Verification items for the finished model (mm, model axes). Face numbers are marked on the shaded views. Give positions to 0.01 mm unless a question says otherwise; leave off trailing zeros. Loops run counter-clockwise (first coordinate to the right, second up) from the corner with the lowest first, then second, coordinate; pieces in that order, holes last. Notation, with made-up numbers: (80.25, 76.25) -> (118.25, 76.25) arc R21 cw to (118.25, 93.25) -> close; hole circle Ø9 at (-35, 55). An arc over 180 degrees is marked (long way). Answer in a Markdown table with one row per item. Add a question column.
Q1. Section check B-B on z = 5. Give the number of separate pieces and of enclosed holes in the cut face, and give its area (3 significant figures).
Q2. Section check C-C on x = 1.5. Enter the section's corners in (y, z).
Q3. Material ranges on probe 1 along Y at (x, z) = (-6, -20); probe 2 along X at (y, z) = (-5.5, 2); probe 3 along Z at (x, y) = (-9, -5.5), recorded low to high.
Q4. Gauge pin test, flat ends, axial feed: P1, Ø1.4, axis at x = 10.5, y = -5, coming from the -Z side; P2, Ø0.6, axis at x = -10.5, y = -3, coming from the -Z side; P3, Ø1.5, axis at x = 13.5, y = -2.5, coming from the +Z side. Record the tip position at first contact, or that the pin passes through.
Q5. Release check for a two-part mould opening along X. For the marked faces 1, 2 and 3 record: pulls with the +X half, pulls with the -X half, needs draft (parallel to the pull), parting line crosses it, or undercut.
Q6. Section check A-A on z = -5.5. Enter the section's corners in (x, y), and give its area (3 significant figures).
```python
from build123d import *

# Parameters (mm, degrees)
F0_R     = 25.4
F1_DEPTH = 6.35
F3_DEPTH = 6.604
F4_DEPTH = 6.604


# Not quite as in the source:
# - the program builds the solid bodies; features that only make, move or delete a surface that nothing else refers to are left out


with BuildPart() as f1:
    # F0 (on Front) → F1 (new body)
    with BuildSketch(Plane.XZ):
        Circle(F0_R)
        with BuildLine():
            Line((-11.384175581, -2.9492764653), (-13.375339268, -2.9492764653))
            Line((-13.375339268, -2.9492764653), (-15.3665029551, -12.3323677108))
            Line((-15.3665029551, -12.3323677108), (-20.4675217554, -12.3323677108))
            Line((-20.4675217554, -12.3323677108), (-15.3022718684, 12.1236185417))
            Line((-15.3022718684, 12.1236185417), (-9.296665264, 12.1236185417))
            add(Edge.make_bspline(
                [(-9.296665264, 12.1236185417), (-5.3303956617, 12.1236185417), (-3.3392319747, 10.4161421542)],
                knots=[0, 0, 0, 1, 1, 1], degree=2))
            add(Edge.make_bspline(
                [(-3.3392319747, 10.4161421542), (-1.3480682877, 8.7086657667), (-1.3480682877, 5.4168225745)],
                knots=[0, 0, 0, 1, 1, 1], degree=2))
            add(Edge.make_bspline(
                [(-1.3480682877, 5.4168225745), (-1.3480682877, 2.7726428396), (-2.7370655371, 0.8751494873)],
                knots=[0, 0, 0, 1, 1, 1], degree=2))
            add(Edge.make_bspline(
                [(-2.7370655371, 0.8751494873), (-4.1260627865, -1.022343865), (-6.738126978, -1.9429894407)],
                knots=[0, 0, 0, 1, 1, 1], degree=2))
            Line((-6.738126978, -1.9429894407), (-2.370413084, -12.3323677108))
            Line((-2.370413084, -12.3323677108), (-7.9264020816, -12.3323677108))
            Line((-7.9264020816, -12.3323677108), (-11.384175581, -2.9492764653))
        make_face(mode=Mode.SUBTRACT)
        with BuildLine():
            Line((9.4748698175, -2.9492764653), (7.4837061305, -2.9492764653))
            Line((7.4837061305, -2.9492764653), (5.4925424435, -12.3323677108))
            Line((5.4925424435, -12.3323677108), (0.3915236432, -12.3323677108))
            Line((0.3915236432, -12.3323677108), (5.5567735302, 12.1236185417))
            Line((5.5567735302, 12.1236185417), (11.5623801345, 12.1236185417))
            add(Edge.make_bspline(
                [(11.5623801345, 12.1236185417), (15.5286497369, 12.1236185417), (17.5198134239, 10.4161421542)],
                knots=[0, 0, 0, 1, 1, 1], degree=2))
            add(Edge.make_bspline(
                [(17.5198134239, 10.4161421542), (19.5109771109, 8.7086657667), (19.5109771109, 5.4168225745)],
                knots=[0, 0, 0, 1, 1, 1], degree=2))
            add(Edge.make_bspline(
                [(19.5109771109, 5.4168225745), (19.5109771109, 2.7726428396), (18.1219798615, 0.8751494873)],
                knots=[0, 0, 0, 1, 1, 1], degree=2))
            add(Edge.make_bspline(
                [(18.1219798615, 0.8751494873), (16.7329826121, -1.022343865), (14.1209184205, -1.9429894407)],
                knots=[0, 0, 0, 1, 1, 1], degree=2))
            Line((14.1209184205, -1.9429894407), (18.4886323146, -12.3323677108))
            Line((18.4886323146, -12.3323677108), (12.932643317, -12.3323677108))
            Line((12.932643317, -12.3323677108), (9.4748698175, -2.9492764653))
        make_face(mode=Mode.SUBTRACT)
    extrude(amount=F1_DEPTH)

    # F0 (on Front) → F3 (join)
    with BuildSketch(Plane.XZ):
        with BuildLine():
            Line((5.4925424435, -12.3323677108), (7.4837061305, -2.9492764653))
            Line((7.4837061305, -2.9492764653), (9.4748698175, -2.9492764653))
            Line((9.4748698175, -2.9492764653), (12.932643317, -12.3323677108))
            Line((12.932643317, -12.3323677108), (18.4886323146, -12.3323677108))
            Line((18.4886323146, -12.3323677108), (14.1209184205, -1.9429894407))
            add(Edge.make_bspline(
                [(18.1219798615, 0.8751494873), (16.7329826121, -1.022343865), (14.1209184205, -1.9429894407)],
                knots=[0, 0, 0, 1, 1, 1], degree=2))
            add(Edge.make_bspline(
                [(19.5109771109, 5.4168225745), (19.5109771109, 2.7726428396), (18.1219798615, 0.8751494873)],
                knots=[0, 0, 0, 1, 1, 1], degree=2))
            add(Edge.make_bspline(
                [(17.5198134239, 10.4161421542), (19.5109771109, 8.7086657667), (19.5109771109, 5.4168225745)],
                knots=[0, 0, 0, 1, 1, 1], degree=2))
            add(Edge.make_bspline(
                [(11.5623801345, 12.1236185417), (15.5286497369, 12.1236185417), (17.5198134239, 10.4161421542)],
                knots=[0, 0, 0, 1, 1, 1], degree=2))
            Line((11.5623801345, 12.1236185417), (5.5567735302, 12.1236185417))
            Line((5.5567735302, 12.1236185417), (0.3915236432, -12.3323677108))
            Line((0.3915236432, -12.3323677108), (5.4925424435, -12.3323677108))
        make_face()
        with BuildLine():
            Line((9.6729156681, 1.2685648932), (8.3668835723, 1.2685648932))
            Line((8.3668835723, 1.2685648932), (9.7746148887, 7.8736616399))
            Line((9.7746148887, 7.8736616399), (11.0110633072, 7.8736616399))
            add(Edge.make_bspline(
                [(13.5133993923, 7.1885300487), (12.7185396947, 7.8736616399), (11.0110633072, 7.8736616399)],
                knots=[0, 0, 0, 1, 1, 1], degree=2))
            add(Edge.make_bspline(
                [(14.30825909, 5.133135275), (14.30825909, 6.5033984574), (13.5133993923, 7.1885300487)],
                knots=[0, 0, 0, 1, 1, 1], degree=2))
            add(Edge.make_bspline(
                [(13.0851921478, 2.2213260123), (14.30825909, 3.1740871313), (14.30825909, 5.133135275)],
                knots=[0, 0, 0, 1, 1, 1], degree=2))
            add(Edge.make_bspline(
                [(9.6729156681, 1.2685648932), (11.8621252057, 1.2685648932), (13.0851921478, 2.2213260123)],
                knots=[0, 0, 0, 1, 1, 1], degree=2))
        make_face(mode=Mode.SUBTRACT)
    extrude(amount=F3_DEPTH)

    # F0 (on Front) → F4 (join)
    with BuildSketch(Plane.XZ):
        with BuildLine():
            Line((-15.3665029551, -12.3323677108), (-13.375339268, -2.9492764653))
            Line((-13.375339268, -2.9492764653), (-11.384175581, -2.9492764653))
            Line((-11.384175581, -2.9492764653), (-7.9264020816, -12.3323677108))
            Line((-7.9264020816, -12.3323677108), (-2.370413084, -12.3323677108))
            Line((-2.370413084, -12.3323677108), (-6.738126978, -1.9429894407))
            add(Edge.make_bspline(
                [(-2.7370655371, 0.8751494873), (-4.1260627865, -1.022343865), (-6.738126978, -1.9429894407)],
                knots=[0, 0, 0, 1, 1, 1], degree=2))
            add(Edge.make_bspline(
                [(-1.3480682877, 5.4168225745), (-1.3480682877, 2.7726428396), (-2.7370655371, 0.8751494873)],
                knots=[0, 0, 0, 1, 1, 1], degree=2))
            add(Edge.make_bspline(
                [(-3.3392319747, 10.4161421542), (-1.3480682877, 8.7086657667), (-1.3480682877, 5.4168225745)],
                knots=[0, 0, 0, 1, 1, 1], degree=2))
            add(Edge.make_bspline(
                [(-9.296665264, 12.1236185417), (-5.3303956617, 12.1236185417), (-3.3392319747, 10.4161421542)],
                knots=[0, 0, 0, 1, 1, 1], degree=2))
            Line((-9.296665264, 12.1236185417), (-15.3022718684, 12.1236185417))
            Line((-15.3022718684, 12.1236185417), (-20.4675217554, -12.3323677108))
            Line((-20.4675217554, -12.3323677108), (-15.3665029551, -12.3323677108))
        make_face()
        with BuildLine():
            Line((-11.1861297305, 1.2685648932), (-12.4921618262, 1.2685648932))
            Line((-12.4921618262, 1.2685648932), (-11.0844305099, 7.8736616399))
            Line((-11.0844305099, 7.8736616399), (-9.8479820913, 7.8736616399))
            add(Edge.make_bspline(
                [(-7.3456460062, 7.1885300487), (-8.1405057038, 7.8736616399), (-9.8479820913, 7.8736616399)],
                knots=[0, 0, 0, 1, 1, 1], degree=2))
            add(Edge.make_bspline(
                [(-6.5507863086, 5.133135275), (-6.5507863086, 6.5033984574), (-7.3456460062, 7.1885300487)],
                knots=[0, 0, 0, 1, 1, 1], degree=2))
            add(Edge.make_bspline(
                [(-7.7738532507, 2.2213260123), (-6.5507863086, 3.1740871313), (-6.5507863086, 5.133135275)],
                knots=[0, 0, 0, 1, 1, 1], degree=2))
            add(Edge.make_bspline(
                [(-11.1861297305, 1.2685648932), (-8.9969201929, 1.2685648932), (-7.7738532507, 2.2213260123)],
                knots=[0, 0, 0, 1, 1, 1], degree=2))
        make_face(mode=Mode.SUBTRACT)
    extrude(amount=F4_DEPTH)


solid = f1.part
```
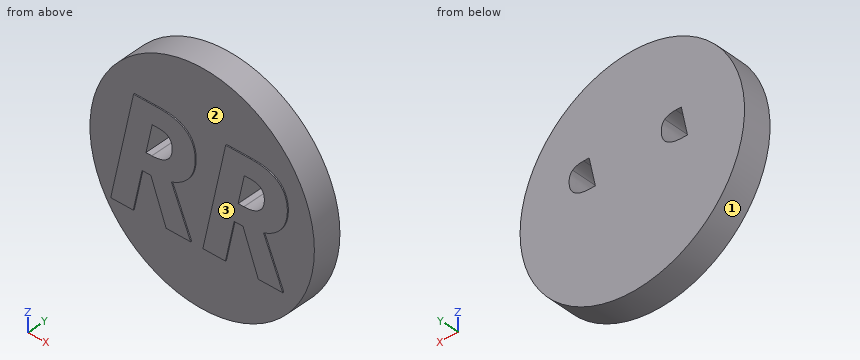
Taken from the geometry:
| question | item | result |
|---|---|---|
| 1 | separate pieces | 3 |
| 1 | enclosed holes | 0 |
| 1 | area | 256 mm² |
| 2 | outline | (-6.6, -12.33) -> (-6.35, -12.33) -> (-6.35, -25.36) -> (0, -25.36) -> (0, 25.36) -> (-6.35, 25.36) -> (-6.35, -7.08) -> (-6.6, -7.08) -> close |
| 3 | probe 1 | y = -6.35 to 0 |
| 3 | probe 2 | x = -25.32 to -12.34, -8.09 to 8.52, 12.77 to 25.32 |
| 3 | probe 3 | z = -23.75 to 1.58, 7.82 to 23.75 |
| 4 | P1 | stops at z = -23.43 |
| 4 | P2 | stops at z = -23.26 |
| 4 | P3 | stops at z = 21.97 |
| 5 | face 1 | parting line crosses it |
| 5 | face 2 | undercut |
| 5 | face 3 | needs draft |
| 6 | outline | (-24.8, -6.35) -> (-19.02, -6.35) -> (-19.02, -6.6) -> (-13.92, -6.6) -> (-13.92, -6.35) -> (-10.44, -6.35) -> (-10.44, -6.6) -> (-5.24, -6.6) -> (-5.24, -6.35) -> (1.83, -6.35) -> (1.83, -6.6) -> (6.94, -6.6) -> (6.94, -6.35) -> (10.41, -6.35) -> (10.41, -6.6) -> (15.62, -6.6) -> (15.62, -6.35) -> (24.8, -6.35) -> (24.8, 0) -> (-24.8, 0) -> close |
| 6 | area | 320 mm² |
